Can you work these out from the model? Positions are in its coordinate system, mm. Round coordinates to 2 decimals unless told otherwise and drop trailing zeros. Write each loop counter-clockwise with the first axis right and the second up, starting at its lowest first coordinate (ties: lowest second). Pieces come first, ordered by that corner, then holes.
Q1. Please list where these lines run through material, in increasing order: line 1 along Y through (x, z) = (-3, 4.25); line 2 along Z through (x, y) = (3.25, -7); line 3 along X through (y, z) = (9, 2.75).
Q2. If we section it at B-B (z = 0): Please give me the cut outline in (x, y), plus the area to 3 significant figures.
Q3. I'm going to push flat-ended pins straight in: pin 1 Ø1 at (x, y) = (-2.5, -27.5) entering from -Z; pin 2 Ø4 at (x, y) = (1, -56.5) entering from -Z; pin 3 Ø6 at (y, z) = (-59.5, -3) entering from -X. Where does each tip first touch, or does it pass through?
Q4. If we section it at C-C (y = -69): Please give me the cut outline in (x, z) (1 decimal), plus the area to 3 significant figures.
Q5. We'd pull the mould along X, two halves only. Please class faces 1 (the flat face through (-3, 0, -4)), 2 (the flat face through (3.1, 12.07, 5.72)), 3 (the cylindrical face through (-3.78, -43.2, -2.9)): +X half, -X half, draft (parallel to the pull), parting line (faces both ways), or undercut.
Q6. If we section it at A-A (y = 7): Please give me the cut outline in (x, z), plus the area to 3 significant figures.
from build123d import *

# Parameters (mm, degrees)
F1_DEPTH = 12.7
F2_R     = 4.7625
F3_DEPTH = 88.9
F4_SIZE  = 1.27


with BuildPart() as f1:
    # F0 (on Front) → F1 (new body)
    with BuildSketch(Plane.XZ):
        Polygon((-0.296798, 8.243551), (-7.287523, 3.864741), (-6.990725, -4.37881), (0.296798, -8.243551), (7.287523, -3.864741), (6.990725, 4.37881), align=None)
    extrude(amount=-F1_DEPTH)

    # F2 (on Front) → F3 (join)
    with BuildSketch(Plane.XZ):
        Circle(F2_R)
    extrude(amount=F3_DEPTH)

    # F4
    f4_edges = [f1.edges().sort_by_distance(p)[0] for p in [
        (-4.7625, -88.9, 0),
        (-7.139124, 12.7, -0.257035),
        (-3.346964, 12.7, -6.31118),
        (3.792161, 12.7, -6.054146),
        (7.139124, 12.7, 0.257035),
        (3.346964, 12.7, 6.31118),
        (-3.792161, 12.7, 6.054146),
    ]]
    chamfer(f4_edges, length=F4_SIZE)


solid = f1.part
A:
1. line 1: y = 0 to 12.7
1. line 2: z = -3.48 to 3.48
1. line 3: x = -7.25 to 7.05
2. outline: (-7.15, 0) - (-4.76, 0) - (-4.76, -87.63) - (-3.49, -88.9) - (3.49, -88.9) - (4.76, -87.63) - (4.76, 0) - (7.15, 0) - (7.15, 11.43) - (5.88, 12.7) - (-5.88, 12.7) - (-7.15, 11.43) - close
2. area: 1,030 mm2
3. pin 1: stops at z = -4.32
3. pin 2: stops at z = -4.76
3. pin 3: stops at x = -4.76
4. outline: circle Ø9.5 at (0, 0)
4. area: 71.3 mm2
5. face 1: draft
5. face 2: +X half
5. face 3: parting line
6. outline: (-7.29, 3.86) - (-6.99, -4.38) - (0.3, -8.24) - (7.29, -3.86) - (6.99, 4.38) - (-0.3, 8.24) - close
6. area: 177 mm2
